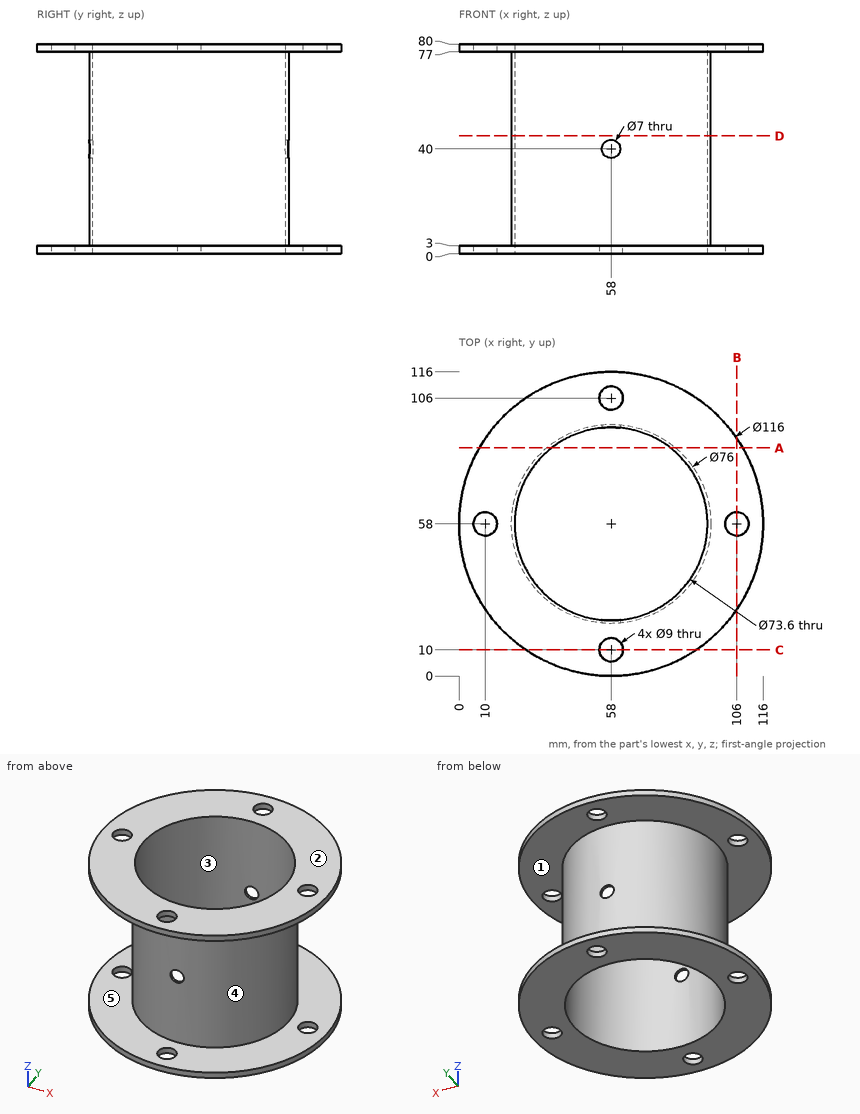
Geometry: see drawing. Coordinates: mm, zero at the bounding-box minimum. A direction names the side the tool comes from. Round coordinates to 2 decimals unless told otherwise and drop trailing zeros. Loops run counter-clockwise (first coordinate to the right, second up) from the corner with the lowest first, then second, coordinate; pieces in that order, holes last. Notation, with made-up numbers: (-6.75, 80.5) -> (46.25, 80.5) arc R34 ccw to (46.25, 111.5) -> close; hole circle Ø4 at (-27, 54). An arc over 180 degrees is marked (long way). Write each question's results on one line, items separated by ' | '.
1. Ray query, line 1 (Y direction, x = 58, z = 78.4); line 2 (Z direction, x = 22.5, y = 80); line 3 (Z direction, x = 58, y = 21). Return the intervals inside material, ascending. Write a range as from..to.
Geometry results:
line 1: 0..5.5, 14.5..21.2, 94.8..101.5, 110.5..116 | line 2: 0..3, 77..80 | line 3: 0..36.5, 43.5..80
2. Mould query, pull axis X, two halves, no side actions, for the marked faces 3, 4 and 5. Classes: +X half, -X half, draft (parallel to the pull), parting line (faces both ways), or undercut.
Geometry results:
face 3: undercut | face 4: parting line | face 5: draft
3. Set-up query: the marked faces 1 and 2. Return all of +Z, -Z, +X, -X, +Y, -Y with unobstructed straight access to the full face (end or side cutting, diameter ignored); none if empty.
Geometry results:
face 1: none | face 2: +Z, +X, -X, +Y, -Y
4. Section D-D (z = 45). Return loops of the section in (x, y).
Geometry results:
outline: circle Ø76 at (58, 58); hole circle Ø73.6 at (58, 58)
5. Section A-A (y = 87). Return loops of the section in (x, z), and give its area (3 significant figures).
Geometry results:
outline: (7.77, 0) -> (35.35, 0) -> (35.35, 80) -> (7.77, 80) -> (7.77, 77) -> (33.44, 77) -> (33.44, 3) -> (7.77, 3) -> close; (80.65, 0) -> (108.23, 0) -> (108.23, 3) -> (82.56, 3) -> (82.56, 77) -> (108.23, 77) -> (108.23, 80) -> (80.65, 80) -> close | area: 612 mm2
6. Section B-B (x = 106). Return loops of the section in (y, z).
Geometry results:
outline: (25.44, 0) -> (53.5, 0) -> (53.5, 3) -> (25.44, 3) -> close; (25.44, 77) -> (53.5, 77) -> (53.5, 80) -> (25.44, 80) -> close; (62.5, 0) -> (90.56, 0) -> (90.56, 3) -> (62.5, 3) -> close; (62.5, 77) -> (90.56, 77) -> (90.56, 80) -> (62.5, 80) -> close
7. First-contact query: P1, Ø3, axis at x = 55.5, z = 48.5, coming from the +Y side; P2, Ø6, axis at y = 39.5, z = 33.5, coming from the +X side; P3, Ø2, axis at y = 89, z = 59.5, coming from the -X side. Flat tips, straight axial feed; report the tip coordinate or a pass-through.
Geometry results:
P1: y = 95.99 | P2: x = 92.7 | P3: x = 34.68
